from build123d import *

# Parameters (mm, degrees)
F0_R     = 59.9535716792
F1_DEPTH = 22.86
F2_R     = 26.8781341555
F3_DEPTH = 22.861
F4_R     = 13.4691567937
F5_DEPTH = 22.861
F7_DEPTH = 25.4
F8_D     = 6.7564


with BuildPart() as f1:
    # F0 (on Front) → F1 (new body)
    with BuildSketch(Plane.XZ):
        with Locations((-19.4891095161, -10.3535922244)):
            Circle(F0_R)
    extrude(amount=F1_DEPTH)

    # F2 (on face) → F3 (cut, through all)
    with BuildSketch(Plane.XZ.offset(22.86)):
        Circle(F2_R)
    extrude(amount=-F3_DEPTH, mode=Mode.SUBTRACT)

    # F4 (on face) → F5 (cut, through all)
    with BuildSketch(Plane.XZ.offset(22.86)):
        with Locations((-43.2526767254, -26.5152305365)):
            Circle(F4_R)
    extrude(amount=-F5_DEPTH, mode=Mode.SUBTRACT)

    # F6 (on Front) → F7 (join)
    with BuildSketch(Plane.XZ):
        with BuildLine():
            Line((125.263456354, 62.0171219158), (32.4955508113, 69.5405378938))
            Line((32.4955508113, 69.5405378938), (33.5459113121, 57.9518266022))
            Line((33.5459113121, 57.9518266022), (41.4141863585, -33.0627560616))
            Line((41.4141863585, -33.0627560616), (187.8204643726, -33.0627560616))
            Line((187.8204643726, -33.0627560616), (175.3908097744, 57.9518266022))
            Line((175.3908097744, 57.9518266022), (139.8324502944, 60.8355861125))
            ThreePointArc((139.8324502944, 60.8355861125), (145.4206878129, 54.9930315803), (147.4552232917, 47.1684224904))
            ThreePointArc((147.4552232917, 47.1684224904), (122.458617796, 33.8177821083), (125.263456354, 62.0171219158))
        make_face()
        with BuildLine():
            Line((139.8324502944, 60.8355861125), (125.263456354, 62.0171219158))
            ThreePointArc((125.263456354, 62.0171219158), (122.458617796, 33.8177821083), (147.4552232917, 47.1684224904))
            ThreePointArc((147.4552232917, 47.1684224904), (145.4206878129, 54.9930315803), (139.8324502944, 60.8355861125))
        make_face()
    extrude(amount=F7_DEPTH)

    # F8 (through all)
    with Locations(Plane(origin=(0, 0, 0), x_dir=(1, 0, 0), z_dir=(0, 1, 0))):
        with Locations((131.3916444778, -47.1684224904)):
            Hole(F8_D / 2)


solid = f1.part
Model file for the job. Use its own axes, mm. A direction names the side the tool comes from. Round coordinates to 2 decimals unless told otherwise and drop trailing zeros. Order: outer loops, then holes, each group sorted by start corner. A loop starts at its lowest first (then second) coordinate and runs counter-clockwise, first axis right, second up.
(1) Pin check, flat tips, straight feed: pin 1 (5 mm diameter, centred on x = 155, y = -9.5, fed in from -Z); pin 2 (2 mm diameter, centred on x = 116.5, z = -33.5, fed in from -Y); pin 3 (10 mm diameter, centred on y = -16.5, z = -16, fed in from +X); pin 4 (6 mm diameter, centred on y = -5.5, z = -19.5, fed in from -X). Stop position of each tip, or through.
(2) Drill centre lines: line 1 (X direction, y = -17.5, z = 8); line 2 (X direction, y = -15.75, z = -33); line 3 (X direction, y = -8.25, z = -23). Where is each one in solid material? Low to high.
(3) Band-saw the part on C-C (y = -3.5). List the corners of the cut face in (x, z), then the cut area to 3 significant figures.
(4) Band-saw the part on A-A (z = -5). List the corners of the cut face in (x, y).
(5) 3-axis set-ups, long thin cutter, end or side, ignore diameter. For faces 4 (the face through (109, -25.4, 19)), 5 (the face through (114, -13, -33.063)): which of +Z, -Z, +X, -X, +Y, -Y reach the whole face in a straight line?
(6) Band-saw the part on D-D (x = 90). List the corners of the cut face in (y, z).
(7) Band-saw the part on B-B (x = 0). List the corners of the cut face in (y, z).
(8) Pull direction X, two halves, no side cores. Call faces 1 (the face through (33.013, -12.522, 63.827)), 2 (the face through (-53.94, -11.59, -34.71)), 3 (the face through (-21, -22.86, -23)): released by +X, released by -X, zero draft, split by the parting line, or undercut.
Verdict:
1. pin 1: stops at z = -33.06
1. pin 2: stops at y = -25.4
1. pin 3: stops at x = 186.17
1. pin 4: stops at x = -79.13
2. line 1: x = -76.56 to -25.66, 25.66 to 37.59, 37.86 to 182.21
2. line 2: x = -75 to -55.06, -31.45 to 36.02, 41.41 to 187.81
2. line 3: x = -78.09 to -56.26, -30.25 to -13.91, 13.91 to 39.12, 40.54 to 186.45
3. outline: (32.5, 69.54) - (33.55, 57.95) - (37.97, 6.75) arc R59.95 ccw (long way) to (40.06, -17.35) - (41.41, -33.06) - (187.82, -33.06) - (175.39, 57.95) - close; hole circle Ø26.94 at (-43.25, -26.52); hole circle Ø53.76 at (0, 0); hole circle Ø6.76 at (131.39, 47.17)
3. area: 22,300 mm2
4. outline: (-79.2, -22.86) - (-26.41, -22.86) - (-26.41, 0) - (-79.2, 0) - close; (26.41, -22.86) - (38.99, -22.86) - (38.99, -25.4) - (183.99, -25.4) - (183.99, 0) - (26.41, 0) - close
5. face 4: +Z, -Z, +X, -X, -Y
5. face 5: -Z, +X, +Y, -Y
6. outline: (-25.4, -33.06) - (0, -33.06) - (0, 64.88) - (-25.4, 64.88) - close
7. outline: (-22.86, -67.05) - (0, -67.05) - (0, -26.88) - (-22.86, -26.88) - close; (-22.86, 26.88) - (0, 26.88) - (0, 46.34) - (-22.86, 46.34) - close
8. face 1: released by -X
8. face 2: undercut
8. face 3: zero draft
